from build123d import *

# Parameters (mm, degrees)
BOSS_EXTRUDE1_DEPTH                             = 3.175
CSK_FOR_M3_FLAT_HEAD_MACHINE_SCREW1_D           = 3.4
CSK_FOR_M3_FLAT_HEAD_MACHINE_SCREW1_CSINK_D     = 6.3
CSK_FOR_M3_FLAT_HEAD_MACHINE_SCREW1_CSINK_ANGLE = 90
SKETCH4_R                                       = 6.9
SKETCH4_R_2                                     = 3.9
SKETCH4_R_3                                     = 3.5
SKETCH4_R_4                                     = 10.1
CUT_EXTRUDE1_DEPTH                              = 4.175


with BuildPart() as part:
    # Sketch1 → Boss-Extrude1 (new body)
    with BuildSketch(Plane(origin=(0, 0, 0), x_dir=(0, 0, -1), z_dir=(1, 0, 0))):
        with BuildLine():
            Line((103.175, 0), (103.175, 3.175))
            Line((103.175, 3.175), (103.175, 47.175))
            Line((103.175, 47.175), (103.175, 50.35))
            Line((103.175, 50.35), (103.175, 70.35))
            Line((103.175, 70.35), (93, 70.35))
            ThreePointArc((93, 70.35), (90.878679656, 69.471320344), (90, 67.35))
            Line((90, 67.35), (90, 53.35))
            ThreePointArc((90, 53.35), (89.121320344, 51.228679656), (87, 50.35))
            Line((87, 50.35), (-87, 50.35))
            ThreePointArc((-87, 50.35), (-89.121320344, 51.228679656), (-90, 53.35))
            Line((-90, 53.35), (-90, 67.35))
            ThreePointArc((-90, 67.35), (-90.878679656, 69.471320344), (-93, 70.35))
            Line((-93, 70.35), (-103.175, 70.35))
            Line((-103.175, 70.35), (-103.175, 50.35))
            Line((-103.175, 50.35), (-103.175, 47.175))
            Line((-103.175, 47.175), (-103.175, 3.175))
            Line((-103.175, 3.175), (-103.175, 0))
            Line((-103.175, 0), (103.175, 0))
        make_face()
    extrude(amount=BOSS_EXTRUDE1_DEPTH)

    # CSK for M3 Flat Head Machine Screw1 (through all)
    with Locations(Plane(origin=(3.175, 0, 0), x_dir=(0, 0, -1), z_dir=(1, 0, 0))):
        with Locations((-75, 8.175), (-65, 8.175), (-95, 65.35)):
            csk_for_m3_flat_head_machine_screw1 = CounterSinkHole(CSK_FOR_M3_FLAT_HEAD_MACHINE_SCREW1_D / 2, CSK_FOR_M3_FLAT_HEAD_MACHINE_SCREW1_CSINK_D / 2, counter_sink_angle=CSK_FOR_M3_FLAT_HEAD_MACHINE_SCREW1_CSINK_ANGLE)

    # Mirror1: CSK for M3 Flat Head Machine Screw1 across plane
    add(csk_for_m3_flat_head_machine_screw1.mirror(Plane.XY), mode=Mode.SUBTRACT)

    # Sketch4 → Cut-Extrude1 (cut, through all)
    with BuildSketch(Plane(origin=(3.175, 0, 0), x_dir=(0, 0, -1), z_dir=(1, 0, 0))):
        with Locations((15, 30.35)):
            Circle(SKETCH4_R)
        with Locations((63.175, 36.35)):
            Circle(SKETCH4_R_2)
        with Locations((50.675, 19.175)):
            Circle(SKETCH4_R_3)
        with Locations((75.675, 19.175)):
            Circle(SKETCH4_R_3)
        with Locations((-15, 30.35)):
            Circle(SKETCH4_R_4)
        with BuildLine():
            ThreePointArc((-62.400909683, 19.212539062), (-63.175, 35.175), (-63.949090317, 19.212539062))
            ThreePointArc((-63.949090317, 19.212539062), (-63.175, 18.4), (-62.400909683, 19.212539062))
        make_face()
    extrude(amount=-CUT_EXTRUDE1_DEPTH, mode=Mode.SUBTRACT)


solid = part.part
Design review of the part built by this model. Coordinates are the model's own, in mm. Coordinates: 2 decimals unless noted, no trailing zeros. Order: outer loops, then holes, each group sorted by start corner. A loop starts at its lowest first (then second) coordinate and runs counter-clockwise, first axis right, second up.
Item 1: Take a section at B-B, the plane y = 30.35. Write out the cut boundary in (x, z) (3 decimals), then the cut area to 3 significant figures.
Item 2: Take a section at A-A, the plane z = 15. Write out the cut boundary in (x, y) (3 decimals).
Item 3: Take a section at D-D, the plane y = 58. Write out the cut boundary in (x, z) (3 decimals).
Item 4: For line 1 (Z direction, x = 1.45, y = 65.35) (3 decimals); line 2 (Y direction, x = 1.5, z = -15); line 3 (Z direction, x = 1.4, y = 59) (3 decimals), list the stretches that pass through material, from the lowest coordinate up.
Item 5: Take a section at C-C, the plane x = 0.75. Count the separate pieces of the cut face and the enclosed holes in it, then the cut area to 3 significant figures.
Item 6: For pin 1 Ø2 at (y, z) = (8.175, 65) entering from +X; pin 2 Ø5.5 at (y, z) = (65.35, -95) entering from +X (3 decimals); pin 3 Ø4 at (y, z) = (8.175, 75) entering from +X (3 decimals); pin 4 Ø1 at (x, z) = (2, 14) entering from +Y, all flat-tipped, find the tip position at first contact; note any pin that passes through.
Item 7: The part is to be moulded in two halves that separate along Y. For faces 1 (the cylindrical face through (0.85, 9.61, -65.91)), 2 (the flat face through (0, 28, 1)), say which applies: pulls with the +Y half, pulls with the -Y half, needs draft (parallel to the pull), parting line crosses it, or undercut.
The answers:
1. outline: (0, -103.175) - (3.175, -103.175) - (3.175, -21.9) - (0, -21.9) - close; (0, -8.1) - (3.175, -8.1) - (3.175, 4.9) - (0, 4.9) - close; (0, 25.1) - (3.175, 25.1) - (3.175, 55.832) - (0, 55.832) - close; (0, 70.518) - (3.175, 70.518) - (3.175, 103.175) - (0, 103.175) - close
1. area: 501 mm2
2. outline: (0, 0) - (3.175, 0) - (3.175, 20.25) - (0, 20.25) - close; (0, 40.45) - (3.175, 40.45) - (3.175, 50.35) - (0, 50.35) - close
3. outline: (0, -103.175) - (3.175, -103.175) - (3.175, -90) - (0, -90) - close; (0, 90) - (3.175, 90) - (3.175, 103.175) - (0, 103.175) - close
4. line 1: z = -103.175 to -96.7, -93.3 to -90, 90 to 93.3, 96.7 to 103.175
4. line 2: y = 0 to 23.45, 37.25 to 50.35
4. line 3: z = -103.175 to -90, 90 to 103.175
5. separate pieces: 1
5. enclosed holes: 12
5. area: 10,100 mm2
6. pin 1: passes through
6. pin 2: stops at x = 2.775
6. pin 3: stops at x = 2.025
6. pin 4: stops at y = 50.35
7. face 1: undercut
7. face 2: needs draft
